Geometry check sheet. Reference: the model listing, model coordinates, mm. A direction names the side the tool comes from. Coordinates: 2 decimals unless noted, no trailing zeros. Write each loop counter-clockwise with the first axis right and the second up, starting at its lowest first coordinate (ties: lowest second). Pieces come first, ordered by that corner, then holes. Notation, with made-up numbers: (-14, 86) -> (38, 86) arc R22 cw to (38, 123) -> close; hole circle Ø5 at (-22, -10.75). An arc over 180 degrees is marked (long way). Use a Markdown table: item, result.
```python
from build123d import *

# Parameters (mm, degrees)
BOSS_EXTRUDE1_DEPTH = 4
SHELL1_T            = -1
BOSS_EXTRUDE2_START = -26
BOSS_EXTRUDE2_DEPTH = 10
BOSS_EXTRUDE3_START = 16
BOSS_EXTRUDE3_DEPTH = 10
BOSS_EXTRUDE5_DEPTH = 2
SKETCH4_3_W         = 9
SKETCH4_3_H         = 21
BOSS_EXTRUDE6_DEPTH = 6
CUT_EXTRUDE1_REACH  = 35.47
FILLET1_R           = 2


with BuildPart() as part:
    # Sketch2 → Boss-Extrude1 (new body)
    with BuildSketch(Plane.XY):
        with BuildLine():
            Line((-3.267949192, 18.5), (3.267949192, 18.5))
            ThreePointArc((3.267949192, 18.5), (4.767949192, 18.098076211), (5.866025404, 17))
            Line((5.866025404, 17), (8.175426481, 13))
            ThreePointArc((8.175426481, 13), (9.273502692, 11.901923789), (10.773502692, 11.5))
            Line((10.773502692, 11.5), (24, 11.5))
            ThreePointArc((24, 11.5), (26.121320344, 10.621320344), (27, 8.5))
            Line((27, 8.5), (27, -8.5))
            ThreePointArc((27, -8.5), (26.121320344, -10.621320344), (24, -11.5))
            Line((24, -11.5), (-24, -11.5))
            ThreePointArc((-24, -11.5), (-26.121320344, -10.621320344), (-27, -8.5))
            Line((-27, -8.5), (-27, 8.5))
            ThreePointArc((-27, 8.5), (-26.121320344, 10.621320344), (-24, 11.5))
            Line((-24, 11.5), (-10.773502692, 11.5))
            ThreePointArc((-10.773502692, 11.5), (-9.273502692, 11.901923789), (-8.175426481, 13))
            Line((-8.175426481, 13), (-5.866025404, 17))
            ThreePointArc((-5.866025404, 17), (-4.767949192, 18.098076211), (-3.267949192, 18.5))
        make_face()
    extrude(amount=BOSS_EXTRUDE1_DEPTH)

    # Shell1
    shell1_openings = [part.faces().sort_by_distance(p)[0] for p in [
        (0, 1.077008716, 4),
    ]]
    offset(amount=SHELL1_T, openings=shell1_openings, kind=Kind.INTERSECTION)

    # Sketch3 → Boss-Extrude2 (add)
    with BuildSketch(Plane(origin=(0, 0, 0), x_dir=(0, 0, -1), z_dir=(1, 0, 0)).offset(BOSS_EXTRUDE2_START)):
        with BuildLine():
            Line((-1, 2.5), (-3.5, 2.5))
            ThreePointArc((-3.5, 2.5), (-6, 5), (-3.5, 7.5))
            Line((-3.5, 7.5), (-1, 7.5))
            Line((-1, 7.5), (-1, 8.5))
            Line((-1, 8.5), (-3.5, 8.5))
            ThreePointArc((-3.5, 8.5), (-7, 5), (-3.5, 1.5))
            Line((-3.5, 1.5), (-1, 1.5))
            Line((-1, 1.5), (-1, 2.5))
        make_face()
    extrude(amount=BOSS_EXTRUDE2_DEPTH)

    # Sketch3<3> → Boss-Extrude3 (add)
    with BuildSketch(Plane(origin=(0, 0, 0), x_dir=(0, 0, -1), z_dir=(1, 0, 0)).offset(BOSS_EXTRUDE3_START)):
        with BuildLine():
            Line((-6.672077255, 6.479163916), (-5.765769468, 6.056545654))
            ThreePointArc((-5.765769468, 6.056545654), (-4.843249021, 7.108478615), (-3.5, 7.5))
            Line((-3.5, 7.5), (-1, 7.5))
            Line((-1, 7.5), (-1, 8.5))
            Line((-1, 8.5), (-3.5, 8.5))
            ThreePointArc((-3.5, 8.5), (-5.380548629, 7.95187006), (-6.672077255, 6.479163916))
        make_face()
        with BuildLine():
            Line((-1, 2.5), (-3.5, 2.5))
            ThreePointArc((-3.5, 2.5), (-5.608478615, 3.656750979), (-5.765769468, 6.056545654))
            Line((-5.765769468, 6.056545654), (-6.672077255, 6.479163916))
            ThreePointArc((-6.672077255, 6.479163916), (-6.45187006, 3.119451371), (-3.5, 1.5))
            Line((-3.5, 1.5), (-1, 1.5))
            Line((-1, 1.5), (-1, 2.5))
        make_face()
    extrude(amount=BOSS_EXTRUDE3_DEPTH)

    # Sketch4 → Boss-Extrude5 (add)
    with BuildSketch(Plane.XY.offset(1)):
        with BuildLine():
            Line((-4.5, 1.5), (-4.5, 7.5))
            Line((-4.5, 7.5), (-10.5, 7.5))
            ThreePointArc((-10.5, 7.5), (-6.257359313, 5.742640687), (-4.5, 1.5))
        make_face()
        with BuildLine():
            Line((10.5, 7.5), (4.5, 7.5))
            Line((4.5, 7.5), (4.5, 1.5))
            ThreePointArc((4.5, 1.5), (6.257359313, 5.742640687), (10.5, 7.5))
        make_face()
    extrude(amount=BOSS_EXTRUDE5_DEPTH)

    # Sketch4<3> → Boss-Extrude6 (add)
    with BuildSketch(Plane.XY.offset(1)):
        Rectangle(SKETCH4_3_W, SKETCH4_3_H)
    extrude(amount=BOSS_EXTRUDE6_DEPTH)

    # Sketch5 → Cut-Extrude1 (cut, up to next)
    with BuildSketch(Plane(origin=(0, 0, 0), x_dir=(1, 0, 0), z_dir=(0, 1, 0)), mode=Mode.PRIVATE) as cut_extrude1_sk1:
        with BuildLine():
            Line((-9.5, -3.5), (-9.5, -1))
            Line((-9.5, -1), (-4.5, -1))
            Line((-4.5, -1), (-4.5, -3.5))
            ThreePointArc((-4.5, -3.5), (-7, -6), (-9.5, -3.5))
        make_face()
    cut_extrude1_tool1 = extrude(cut_extrude1_sk1.sketch, amount=-CUT_EXTRUDE1_REACH, mode=Mode.PRIVATE) & part.part
    # Sketch5 → Cut-Extrude1 (cut, up to next)
    with BuildSketch(Plane(origin=(0, 0, 0), x_dir=(1, 0, 0), z_dir=(0, 1, 0)), mode=Mode.PRIVATE) as cut_extrude1_sk2:
        with BuildLine():
            Line((4.5, -3.5), (4.5, -1))
            Line((4.5, -1), (9.5, -1))
            Line((9.5, -1), (9.5, -3.5))
            ThreePointArc((9.5, -3.5), (7, -6), (4.5, -3.5))
        make_face()
    cut_extrude1_tool2 = extrude(cut_extrude1_sk2.sketch, amount=-CUT_EXTRUDE1_REACH, mode=Mode.PRIVATE) & part.part
    add(cut_extrude1_tool1.solids().sort_by_distance((-7, 0, 3.266625))[0], mode=Mode.SUBTRACT)
    add(cut_extrude1_tool2.solids().sort_by_distance((7, 0, 3.266625))[0], mode=Mode.SUBTRACT)

    # Fillet1
    # the kernel refuses this fillet: 2 mm, written as the material it takes off along each edge
    with BuildSketch(Plane(origin=(27, 8.5, 0), x_dir=(0, 0, 1), z_dir=(0, -1, 0)), Plane(origin=(-27, -8.5, 0), x_dir=(0, 0, 1), z_dir=(0, 1, 0))) as fillet1_piece_1:
        with BuildLine():
            CenterArc((FILLET1_R, FILLET1_R), FILLET1_R, 180, 90)
            Line((0, FILLET1_R), (0, 0))
            Line((0, 0), (FILLET1_R, 0))
        make_face()
    extrude(amount=17, mode=Mode.SUBTRACT)
    with BuildSketch(Plane(origin=(24, 8.5, 0), x_dir=(0, 1, 0), z_dir=(-1, 0, 0))) as fillet1_piece_2:
        with BuildLine():
            CenterArc((3 - FILLET1_R, -FILLET1_R), FILLET1_R, 0, 90)
            Line((3 - FILLET1_R, 0), (3, 0))
            Line((3, 0), (3, -FILLET1_R))
        make_face()
    revolve(axis=Axis((24, 8.5, 0), (0, 0, -1)), revolution_arc=90, mode=Mode.SUBTRACT)
    with BuildSketch(Plane(origin=(10.773502692, 11.5, 0), x_dir=(0, 0, 1), z_dir=(1, 0, 0)), Plane(origin=(-24, 11.5, 0), x_dir=(0, 0, 1), z_dir=(1, 0, 0))) as fillet1_piece_3:
        with BuildLine():
            CenterArc((FILLET1_R, FILLET1_R), FILLET1_R, 180, 90)
            Line((0, FILLET1_R), (0, 0))
            Line((0, 0), (FILLET1_R, 0))
        make_face()
    extrude(amount=13.226497308, mode=Mode.SUBTRACT)
    with BuildSketch(Plane(origin=(10.773502692, 14.5, 0), x_dir=(-0.8660254037844389, -0.49999999999999956, 0), z_dir=(-0.49999999999999956, 0.8660254037844389, 0))) as fillet1_piece_4:
        with BuildLine():
            CenterArc((3 + FILLET1_R, FILLET1_R), FILLET1_R, 180, 90)
            Line((3 + FILLET1_R, 0), (3, 0))
            Line((3, 0), (3, FILLET1_R))
        make_face()
    revolve(axis=Axis((10.773502692, 14.5, 0), (0, 0, 1)), revolution_arc=60, mode=Mode.SUBTRACT)
    with BuildSketch(Plane(origin=(5.866025404, 17, 0), x_dir=(0, 0, 1), z_dir=(0.500000000000004, -0.8660254037844364, 0)), Plane(origin=(-8.175426481, 13, 0), x_dir=(0, 0, 1), z_dir=(0.5000000000000043, 0.8660254037844362, 0))) as fillet1_piece_5:
        with BuildLine():
            CenterArc((FILLET1_R, FILLET1_R), FILLET1_R, 180, 90)
            Line((0, FILLET1_R), (0, 0))
            Line((0, 0), (FILLET1_R, 0))
        make_face()
    extrude(amount=4.618802154, mode=Mode.SUBTRACT)
    with BuildSketch(Plane(origin=(3.267949192, 15.5, 0), x_dir=(0, 1, 0), z_dir=(-1, 0, 0))) as fillet1_piece_6:
        with BuildLine():
            CenterArc((3 - FILLET1_R, -FILLET1_R), FILLET1_R, 0, 90)
            Line((3 - FILLET1_R, 0), (3, 0))
            Line((3, 0), (3, -FILLET1_R))
        make_face()
    revolve(axis=Axis((3.267949192, 15.5, 0), (0, 0, -1)), revolution_arc=60, mode=Mode.SUBTRACT)
    with BuildSketch(Plane(origin=(-3.267949192, 18.5, 0), x_dir=(0, 0, 1), z_dir=(1, 0, 0))) as fillet1_piece_7:
        with BuildLine():
            CenterArc((FILLET1_R, FILLET1_R), FILLET1_R, 180, 90)
            Line((0, FILLET1_R), (0, 0))
            Line((0, 0), (FILLET1_R, 0))
        make_face()
    extrude(amount=6.535898385, mode=Mode.SUBTRACT)
    with BuildSketch(Plane(origin=(-3.267949192, 15.5, 0), x_dir=(-0.8660254037844407, 0.4999999999999964, 0), z_dir=(-0.4999999999999964, -0.8660254037844407, 0))) as fillet1_piece_8:
        with BuildLine():
            CenterArc((3 - FILLET1_R, -FILLET1_R), FILLET1_R, 0, 90)
            Line((3 - FILLET1_R, 0), (3, 0))
            Line((3, 0), (3, -FILLET1_R))
        make_face()
    revolve(axis=Axis((-3.267949192, 15.5, 0), (0, 0, -1)), revolution_arc=60, mode=Mode.SUBTRACT)
    with BuildSketch(Plane(origin=(-10.773502692, 14.5, 0), x_dir=(0, -1, 0), z_dir=(-1, 0, 0))) as fillet1_piece_9:
        with BuildLine():
            CenterArc((3 + FILLET1_R, FILLET1_R), FILLET1_R, 180, 90)
            Line((3, FILLET1_R), (3, 0))
            Line((3, 0), (3 + FILLET1_R, 0))
        make_face()
    revolve(axis=Axis((-10.773502692, 14.5, 0), (0, 0, 1)), revolution_arc=60, mode=Mode.SUBTRACT)
    with BuildSketch(Plane(origin=(-24, 8.5, 0), x_dir=(-1, 0, 0), z_dir=(0, -1, 0))) as fillet1_piece_10:
        with BuildLine():
            CenterArc((3 - FILLET1_R, -FILLET1_R), FILLET1_R, 0, 90)
            Line((3, -FILLET1_R), (3, 0))
            Line((3, 0), (3 - FILLET1_R, 0))
        make_face()
    revolve(axis=Axis((-24, 8.5, 0), (0, 0, -1)), revolution_arc=90, mode=Mode.SUBTRACT)
    with BuildSketch(Plane(origin=(-24, -8.5, 0), x_dir=(0, -1, 0), z_dir=(1, 0, 0))) as fillet1_piece_11:
        with BuildLine():
            CenterArc((3 - FILLET1_R, -FILLET1_R), FILLET1_R, 0, 90)
            Line((3 - FILLET1_R, 0), (3, 0))
            Line((3, 0), (3, -FILLET1_R))
        make_face()
    revolve(axis=Axis((-24, -8.5, 0), (0, 0, -1)), revolution_arc=90, mode=Mode.SUBTRACT)
    with BuildSketch(Plane(origin=(24, -11.5, 0), x_dir=(0, 0, 1), z_dir=(-1, 0, 0))) as fillet1_piece_12:
        with BuildLine():
            CenterArc((FILLET1_R, FILLET1_R), FILLET1_R, 180, 90)
            Line((0, FILLET1_R), (0, 0))
            Line((0, 0), (FILLET1_R, 0))
        make_face()
    extrude(amount=48, mode=Mode.SUBTRACT)
    with BuildSketch(Plane(origin=(24, -8.5, 0), x_dir=(1, 0, 0), z_dir=(0, 1, 0))) as fillet1_piece_13:
        with BuildLine():
            CenterArc((3 - FILLET1_R, -FILLET1_R), FILLET1_R, 0, 90)
            Line((3 - FILLET1_R, 0), (3, 0))
            Line((3, 0), (3, -FILLET1_R))
        make_face()
    revolve(axis=Axis((24, -8.5, 0), (0, 0, -1)), revolution_arc=90, mode=Mode.SUBTRACT)


solid = part.part
```
Item 1: Section check B-B on z = 4.5. Record the boundary of the cut face in (x, y), then the cut area to 3 significant figures.
Answer block:
| item | result |
|---|---|
| outline | (-26, 1.65) -> (-16, 1.65) -> (-16, 2.71) -> (-26, 2.71) -> close; (-26, 7.29) -> (-16, 7.29) -> (-16, 8.35) -> (-26, 8.35) -> close; (-4.5, -10.5) -> (4.5, -10.5) -> (4.5, 10.5) -> (-4.5, 10.5) -> close; (16, 1.65) -> (26, 1.65) -> (26, 2.71) -> (16, 2.71) -> close; (16, 7.29) -> (26, 7.29) -> (26, 8.35) -> (16, 8.35) -> close |
| area | 232 mm^2 |
Item 2: Mould release check, pull along Y, two halves, no side actions. Record for faces 5 (the flat face through (-17, -11.5, 3)), 6 (the flat face through (27, 0, 3)), 7 (the cylindrical face through (25.4, 9.93, 2.48)): +Y half, -Y half, draft (parallel to the pull), parting line (faces both ways), or undercut.
Answer block:
| item | result |
|---|---|
| face 5 | -Y half |
| face 6 | draft |
| face 7 | undercut |
Item 3: Section check A-A on x = 0.5. Record the boundary of the cut face in (y, z), then the cut area to 3 significant figures.
Answer block:
| item | result |
|---|---|
| outline | (-11.5, 2) arc R2 ccw to (-9.5, 0) -> (16.5, 0) arc R2 ccw to (18.5, 2) -> (18.5, 4) -> (17.5, 4) -> (17.5, 1) -> (10.5, 1) -> (10.5, 7) -> (-10.5, 7) -> (-10.5, 4) -> (-11.5, 4) -> close |
| area | 160 mm^2 |
Item 4: Thickness scan on L1, parallel to X at y = 1, z = 3.25; L2, parallel to Y at x = -13, z = 3.75; L3, parallel to Y at x = 17, z = 2.25. Record the ranges inside material, lowest first. Write a range as [from, to].
Answer block:
| item | result |
|---|---|
| L1 | x = [-27, -26], [-4.5, 4.5], [26, 27] |
| L2 | y = [-11.5, -10.5], [10.5, 11.5] |
| L3 | y = [-11.5, -10.5], [1.5, 2.5], [7.5, 8.5], [10.5, 11.5] |
Item 5: Depth check by flat-ended pin: P1, Ø2.5, axis at y = 6, z = 6, coming from the -X side; P2, Ø2, axis at y = -6, z = 6, coming from the -X side; P3, Ø5, axis at x = -18.5, y = 12, coming from the +Z side. Enter the tip coordinate at first touch or a pass-through.
Answer block:
| item | result |
|---|---|
| P1 | stops at x = -26 |
| P2 | stops at x = -4.5 |
| P3 | stops at z = 4 |
Item 6: Section check D-D on x = 22.5. Record the boundary of the cut face in (y, z), then the cut area to 3 significant figures.
Answer block:
| item | result |
|---|---|
| outline | (-11.5, 2) arc R2 ccw to (-9.5, 0) -> (9.5, 0) arc R2 ccw to (11.5, 2) -> (11.5, 4) -> (10.5, 4) -> (10.5, 1) -> (8.5, 1) -> (8.5, 3.5) arc R3.5 ccw to (1.5, 3.5) -> (1.5, 1) -> (-10.5, 1) -> (-10.5, 4) -> (-11.5, 4) -> close; hole (2.5, 1) -> (7.5, 1) -> (7.5, 3.5) arc R2.5 ccw to (2.5, 3.5) -> close |
| area | 41.7 mm^2 |
Item 7: Tool access check on faces 1 (the flat face through (26, 5, 2)), 2 (the flat face through (21, 8.5, 2)), 3 (the flat face through (-26, 5, 6.2)), 4 (the flat face through (0, -11, 4)). Record the directions out of +Z, -Z, +X, -X, +Y, -Y that give a thin tool (end or side, any length) a straight path to the whole face; none if there is none.
Answer block:
| item | result |
|---|---|
| face 1 | none |
| face 2 | +Z |
| face 3 | +Z, -X, +Y, -Y |
| face 4 | +Z, +X, -X, -Y |
Item 8: Section check C-C on y = 5. Record the boundary of the cut face in (x, z), then the cut area to 3 significant figures.
Answer block:
| item | result |
|---|---|
| outline | (-27, 2) arc R2 ccw to (-25, 0) -> (25, 0) arc R2 ccw to (27, 2) -> (27, 4) -> (26, 4) -> (26, 1) -> (5.63, 1) -> (5.63, 3) -> (4.5, 3) -> (4.5, 7) -> (-4.5, 7) -> (-4.5, 3) -> (-5.63, 3) -> (-5.63, 1) -> (-26, 1) -> (-26, 4) -> (-27, 4) -> close; (-26, 6) -> (-16, 6) -> (-16, 7) -> (-26, 7) -> close; (16, 6) -> (26, 6) -> (26, 7) -> (16, 7) -> close |
| area | 137 mm^2 |
